For this review, take the finished solid that the model builds, in its own axes (mm). A direction names the side the tool comes from. Coordinates: 2 decimals unless noted, no trailing zeros. Loops run counter-clockwise (first coordinate to the right, second up) from the corner with the lowest first, then second, coordinate; pieces in that order, holes last. Notation, with made-up numbers: (88, 88.25) -> (132, 88.25) arc R19 ccw to (132, 92.25) -> close; hole circle Ø8 at (-27, 71). An arc over 180 degrees is marked (long way). Answer in a Markdown table with one row per item.
from build123d import *

# Parameters (mm, degrees)
F1_DEPTH = 160
F2_R     = 50
F3_DEPTH = 504
F4_R     = 50
F5_DEPTH = 50


with BuildPart() as f1:
    # F0 (on Top) → F1 (new body)
    with BuildSketch(Plane.XY):
        with BuildLine():
            Line((-43.5, -100), (43.5, -100))
            Line((43.5, -100), (43.5, 100))
            Line((43.5, 100), (-43.5, 100))
            ThreePointArc((-43.5, 100), (-143.5, 0), (-43.5, -100))
        make_face()
    extrude(amount=F1_DEPTH)

    # F2 (on face) → F3 (cut)
    with BuildSketch(Plane.XY.offset(160)):
        with Locations((-43.5, 0)):
            Circle(F2_R)
    extrude(amount=-F3_DEPTH, mode=Mode.SUBTRACT)

    # F4 (on face) → F5 (join)
    with BuildSketch(Plane.YZ.offset(43.5)):
        with Locations((0, 80)):
            Circle(F4_R)
    extrude(amount=F5_DEPTH)


solid = f1.part
Item 1: Insertion check: pin 1 (8 mm diameter, centred on x = -51.5, z = 124, fed in from -Y); pin 2 (3 mm diameter, centred on x = 55, y = 22, fed in from +Z); pin 3 (2 mm diameter, centred on x = 51, y = -21, fed in from +Z). Each pin has a flat end and moves straight along its axis. Give the tip position at first contact, or say it passes through.
Worked answers:
| item | result |
|---|---|
| pin 1 | y = -99.92 |
| pin 2 | z = 125.6 |
| pin 3 | z = 125.83 |
Item 2: For L1, parallel to Y at x = -43.5, z = 62.5; L2, parallel to Y at x = -71, z = 73; L3, parallel to X at y = 17, z = 25, list the stretches that pass through material, from the lowest coordinate up.
Worked answers:
| item | result |
|---|---|
| L1 | -100 to -50, 50 to 100 |
| L2 | -96.14 to -41.76, 41.76 to 96.14 |
| L3 | -142.04 to -90.52, 3.52 to 43.5 |
Item 3: For faces 5 (the cylindrical face through (68.15, 23.07, 35.64)), 6 (the flat face through (11, 1, 160)), list the 3-axis set-ups (+Z, -Z, +X, -X, +Y, -Y) from which the entire face can be reached by the end or side of a thin tool; tool diameter is ignored.
Worked answers:
| item | result |
|---|---|
| face 5 | +X |
| face 6 | +Z, +X, -X, +Y, -Y |
Item 4: Take a section at B-B, the plane z = 50. State the section outline as (x, y) points.
Worked answers:
| item | result |
|---|---|
| outline | (-43.5, -100) -> (43.5, -100) -> (43.5, -40) -> (93.5, -40) -> (93.5, 40) -> (43.5, 40) -> (43.5, 100) -> (-43.5, 100) arc R100 ccw to start; hole circle Ø100 at (-43.5, 0) |
Item 5: Take a section at C-C, the plane x = -8. State the section outline as (y, z) points, and give its area (3 significant figures).
Worked answers:
| item | result |
|---|---|
| outline | (-100, 0) -> (-35.21, 0) -> (-35.21, 160) -> (-100, 160) -> close; (35.21, 0) -> (100, 0) -> (100, 160) -> (35.21, 160) -> close |
| area | 20,700 mm² |
Item 6: The part is to be moulded in two halves that separate along X. For faces 1 (the flat face through (43.5, -1, 26)), 2 (the cylindrical face through (-80.352, 33.792, 81.12)), 3 (the flat face through (11, 1, 0)), 4 (the cylindrical face through (-143.476, 2.199, 78.88)), say which applies: +X half, -X half, draft (parallel to the pull), parting line (faces both ways), or undercut.
Worked answers:
| item | result |
|---|---|
| face 1 | +X half |
| face 2 | undercut |
| face 3 | draft |
| face 4 | -X half |
Item 7: Take a section at D-D, the plane z = 80. State the section outline as (x, y) points.
Worked answers:
| item | result |
|---|---|
| outline | (-43.5, -100) -> (43.5, -100) -> (43.5, -50) -> (93.5, -50) -> (93.5, 50) -> (43.5, 50) -> (43.5, 100) -> (-43.5, 100) arc R100 ccw to start; hole circle Ø100 at (-43.5, 0) |
Item 8: Take a section at A-A, the plane y = 0. State the section outline as (x, z) points, and give its area (3 significant figures).
Worked answers:
| item | result |
|---|---|
| outline | (-143.5, 0) -> (-93.5, 0) -> (-93.5, 160) -> (-143.5, 160) -> close; (6.5, 0) -> (43.5, 0) -> (43.5, 30) -> (93.5, 30) -> (93.5, 130) -> (43.5, 130) -> (43.5, 160) -> (6.5, 160) -> close |
| area | 18,900 mm² |
